The figure shows three views and two pictorial views of one solid part (mm, origin at its lowest corner). Answer the questions. Coordinates: 2 decimals unless noted, no trailing zeros. Order: outer loops, then holes, each group sorted by start corner. A loop starts at its lowest first (then second) coordinate and runs counter-clockwise, first axis right, second up. Notation, with made-up numbers: (0, 50) -> (19, 50) arc R13 cw to (19, 61) -> close; hole circle Ø2 at (-27.75, 68.25). An arc over 180 degrees is marked (long way). Write item = value, one per line. Start each with the question number.
Q1. The part is cut by section A-A, the plane y = 80. Determine the outline of the cut face in (x, z).
Q2. Flat-ended cylindrical pins translate along their axes: pin 1 (4.5 mm diameter, centred on y = 38, z = 6.5, fed in from +X); pin 2 (4.5 mm diameter, centred on x = 16, z = 6, fed in from -Y); pin 3 (1.5 mm diameter, centred on x = 34, z = 6, fed in from +Y); pin 4 (2 mm diameter, centred on y = 46, z = 5.5, fed in from -X). Find the tip coordinate at first contact, or state that the pin passes through.
Q3. The part is cut by section B-B, the plane z = 7. Determine the outline of the cut face in (x, y).
Q4. Straight lines are drawn through the part: L1, parallel to Y at x = 8, z = 4.5; L2, parallel to X at y = 58, z = 5; L3, parallel to Y at x = 4, z = 5.5. For each, find the intervals that lie inside material, in ascending order. Write a range as from..to.
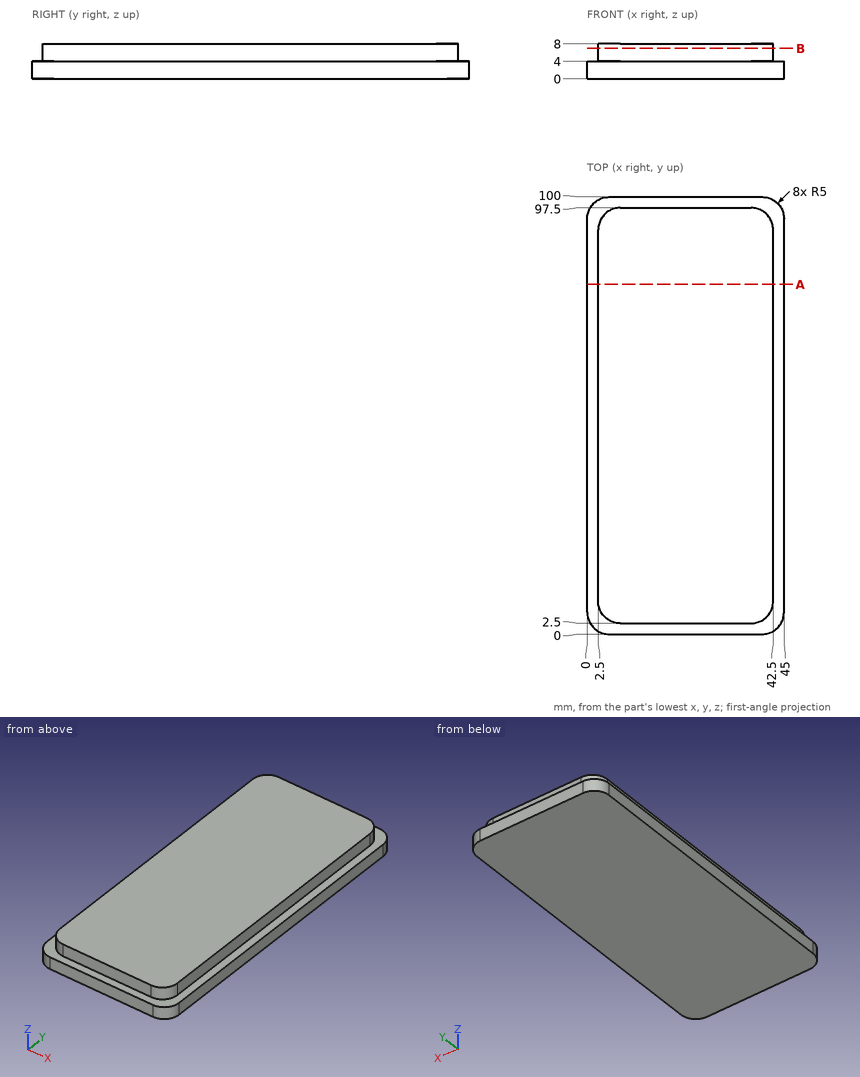
Model answer:
q1.outline = (0, 0) -> (45, 0) -> (45, 4) -> (42.5, 4) -> (42.5, 8) -> (2.5, 8) -> (2.5, 4) -> (0, 4) -> close
q2.pin_1 = 42.5
q2.pin_2 = 0
q2.pin_3 = 97.5
q2.pin_4 = 2.5
q3.outline = (2.5, 7.5) arc R5 ccw to (7.5, 2.5) -> (37.5, 2.5) arc R5 ccw to (42.5, 7.5) -> (42.5, 92.5) arc R5 ccw to (37.5, 97.5) -> (7.5, 97.5) arc R5 ccw to (2.5, 92.5) -> close
q4.L1 = 2.5..97.5
q4.L2 = 2.5..42.5
q4.L3 = 3.93..96.07
